Part model, mm, in its own coordinate system. Face numbers are marked on the shaded views. Round coordinates to 2 decimals unless told otherwise and drop trailing zeros. Loops run counter-clockwise (first coordinate to the right, second up) from the corner with the lowest first, then second, coordinate; pieces in that order, holes last. Notation, with made-up numbers: M 44,82 L 76,82 A17 ccw 76,94 Z; hole C -3.5,28 d4. An arc over 180 degrees is marked long. Put each result on its own line as item: value. Start each with the question number.
1) Slice it at C-C on x = 97. Give the cut face in (y, z).
2) Slice it at A-A on y = -75. Give the cut face in (x, z), then the cut area to 3 significant figures.
3) Slice it at B-B on z = 558.5. Give the cut face in (x, y).
4) Pull direction X, two halves, no side cores. Call the marked faces 1, 2 and 3: +X half, -X half, draft (parallel to the pull), parting line (faces both ways), or undercut.
5) Slice it at D-D on z = 704. Give the cut face in (x, y), then the cut area to 3 significant figures.
6) Drop flat-ended pins along their axis: pin 1 Ø6 at (x, y) = (307, -46.5) entering from +Z; pin 2 Ø10 at (y, z) = (-132.5, 822.5) entering from -X; pin 3 Ø6 at (x, y) = (138, -55) entering from -Z; pin 4 Ø6 at (y, z) = (-37.5, 229.5) entering from -X. Give the stop position or say it passes through.
7) Probe line 1 along X through (y, z) = (-75, 593); line 2 along Y through (x, z) = (75, 238); line 3 along Z through (x, y) = (441.5, -75). List the from-to ranges inside material, lowest first.
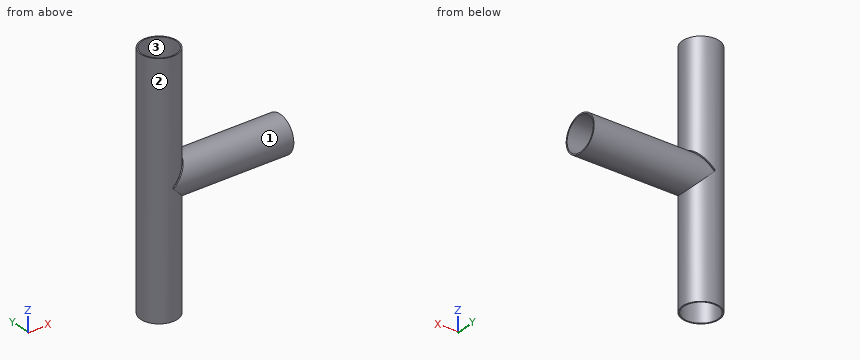
Autodesk Inventor part; units mm, degrees
ref_plane "YZ Plane" through (0, 0, 0) normal (1, 0, 0) x (0, 1, 0)
ref_plane "XZ Plane" through (0, 0, 0) normal (0, 1, 0) x (-1, 0, 0)
ref_plane "XY Plane" through (0, 0, 0) normal (0, 0, 1) x (1, 0, 0)
sketch "Эскиз1" plane through (0, 0, 0) normal (0, 0, 1) x (1, 0, 0)
  line L0 (0, 0) -> (150, 0)
  line L1 (150, 0) -> (150, -150)
  line L2 (150, -150) -> (0, -150)
  line L3 (0, -150) -> (0, 0)
  dimension "d0" = 150
  dimension "d1" = 150
extrude "Выдавливание1" add sketch "Эскиз1" along normal blind 1000
sketch "Эскиз2" plane through (150, -150, 0) normal (1, 0, 0) x (0, 0, -1)
  line L0 (0, 0) -> (-1000, 0)
  line L1 (0, 150) -> (-1000, 150)
  line L2 (-575, 0) -> (-425, 0)
  line L3 (-425, 0) -> (-425, 150)
  line L4 (-425, 150) -> (-575, 150)
  line L5 (-575, 150) -> (-575, 0)
  point P0 (-500, 0)
  point P1 (-500, 0)
  point P2 (-425, 0)
  dimension "d4" = 150
  dimension "d5" = 0
extrude "Выдавливание2" add sketch "Эскиз2" along normal blind 425
sketch "Эскиз3" plane through (0, 0, 0) normal (0, 1, 0) x (1, 0, 0)
  line L0 (150, -425) -> (575, -425)
  line L1 (150, -575) -> (575, -575)
  line L2 (150, -425) -> (150, -575)
  line L3 (150, -500) -> (0, -500)
  line L4 (0, 0) -> (0, -1000)
  line L5 (75, -500) -> (150, -575)
  line L6 (80, -500) -> (155, -575)
  line L7 (70, -500) -> (150, -580)
  line L8 (150, -575) -> (150, -1000)
  circle A0 centre (77.5, -502.5) radius 3.5355
  point P0 (150, -570)
  point P1 (75, -505)
  dimension "d8" = 5
  dimension "d9" = 5
extrude "Выдавливание3" cut sketch "Эскиз3" against normal blind 200 contours L2 L6 L1 | L5 A0 L6 L2 | L8 L7 A0 L5 | A0 L5 | L5 L3 A0 | L3 A0
fillet "Сопряжение1" radius 75 10 edges at (365, 0, 575) (362.5, 0, 425) (365, -150, 575) (362.5, -150, 425) (150, -150, 212.5) (150, 0, 212.5) (150, 0, 790) (150, -150, 790) (0, -150, 500) (0, 0, 500)
sketch "Эскиз4" plane through (75, -75, 1000) normal (0, 0, 1) x (1, 0, 0)
  line L0 (0, 75) -> (0, -75)
  circle A0 centre (0, 0) radius 70
  point P0 (-75, 75)
  dimension "d13" = 140
extrude "Выдавливание4" cut sketch "Эскиз4" against normal blind 1010
sketch "Эскиз5" plane through (575, -75, 500) normal (1, 0, 0) x (0, 0, -1)
  circle A0 centre (0, 0) radius 70
  point P0 (500, 75)
  dimension "d16" = 140
extrude "Выдавливание5" cut sketch "Эскиз5" against normal blind 500
properties part number "вставка в трубу" material "Полистирол, высокопрочный"
Recorded:
1. outline: M -148.05,517 A75 ccw -146.7,478 L -146.7,0 L -141.45,0 L -141.45,478 A70 cw -142.9,517 Z; M -146.7,527 L -141.45,527 L -141.45,1000 L -146.7,1000 Z; M -8.55,0 L -3.3,0 L -3.3,478 A75 ccw -1.95,517 L -7.1,517 A70 cw -8.55,478 Z; M -8.55,527 L -3.3,527 L -3.3,1000 L -8.55,1000 Z
2. outline: M 0,0 L 5,0 L 5,1000 L 0,1000 Z; M 145,0 L 150,0 L 150,425 L 575,425 L 575,430 L 145,430 Z; M 145,575 L 150,580 L 150,1000 L 145,1000 Z; M 150,570 L 575,570 L 575,575 L 155,575 Z
2. area: 13,500 mm2
3. outline: M 128.5,-127.56 L 128.5,-120.14 A70 cw long 128.5,-29.86 L 128.5,-22.44 A75 ccw long Z; M 138.5,-121.93 L 575,-121.93 L 575,-113.44 L 138.5,-113.44 Z; M 138.5,-36.56 L 575,-36.56 L 575,-28.07 L 138.5,-28.07 Z
4. face 1: draft
4. face 2: parting line
4. face 3: undercut
5. outline: C 75,-75 d150; hole C 75,-75 d140
5. area: 2,280 mm2
6. pin 1: stops at z = 570.53
6. pin 2: stops at x = 21.44
6. pin 3: passes through
6. pin 4: stops at x = 8.41
7. line 1: x = 0 to 5, 145 to 150
7. line 2: y = -150 to -145, -5 to 0
7. line 3: z = 425 to 430, 570 to 575
